The listing builds one solid part. Answer for the finished solid, in the listing's coordinates (mm). A direction names the side the tool comes from. Round coordinates to 2 decimals unless told otherwise and drop trailing zeros. Loops run counter-clockwise (first coordinate to the right, second up) from the corner with the lowest first, then second, coordinate; pieces in that order, holes last. Notation, with made-up numbers: (74.5, 1) - (125.5, 1) arc R16 cw to (125.5, 28) - close; hole circle Ø2 at (-7, 19.25). An arc over 180 degrees is marked (long way). One line per item, written item: value.
```python
from build123d import *

# Parameters (mm, degrees)
SKETCH1_R         = 50.8
EXTRUDE1_DEPTH    = 7.62
SKETCH2_R         = 21.463
EXTRUDE2_DEPTH    = 24.892
SKETCH3_R         = 3.175
EXTRUDE3_DEPTH    = 8.62
CIRPATTERN1_COUNT = 4
FILLET1_R         = 1.154545455
SKETCH4_W         = 79.017488084
SKETCH4_H         = 12.7


with BuildPart() as part:
    # Sketch1 → Extrude1 (new body)
    with BuildSketch(Plane.XY):
        Circle(SKETCH1_R)
    extrude(amount=EXTRUDE1_DEPTH)

    # Sketch2 → Extrude2 (add)
    with BuildSketch(Plane.XY.offset(7.62)):
        Circle(SKETCH2_R)
    extrude(amount=EXTRUDE2_DEPTH)

    # Sketch3 → Extrude3 (cut, through all)
    with BuildSketch(Plane.XY.offset(7.62)):
        with Locations((0, 36.1315)):
            Circle(SKETCH3_R)
    extrude3 = extrude(amount=-EXTRUDE3_DEPTH, mode=Mode.SUBTRACT)

    # CirPattern1: Extrude3 ×4 about axis
    cirpattern1_axis = Axis((0, 0, 0), (0, 0, 1))
    for i in range(1, CIRPATTERN1_COUNT):
        add(extrude3.rotate(cirpattern1_axis, i * 360 / CIRPATTERN1_COUNT), mode=Mode.SUBTRACT)

    # Fillet1
    fillet1_edges = [part.edges().sort_by_distance(p)[0] for p in [
        (-50.8, 0, 7.62),
        (-21.463, 0, 7.62),
        (-21.463, 0, 32.512),
    ]]
    fillet(fillet1_edges, radius=FILLET1_R)

    # Sketch4 → Cut-Revolve1 (revolve, cut)
    with BuildSketch(Plane(origin=(0, 0, 63.5), x_dir=(0, 0, -1), z_dir=(1, 0, 0))):
        with Locations((39.507700489, 6.35)):
            Rectangle(SKETCH4_W, SKETCH4_H)
    revolve(axis=Axis((0, 0, -15.516444531), (0, 0, 1)), mode=Mode.SUBTRACT)


solid = part.part
```
1) For faces 1 (the flat face through (10, -21, 7.62)), 2 (the cylindrical face through (0.688, -33.032, 3.863)), determine the directions among +Z, -Z, +X, -X, +Y, -Y from which every point of the face is accessible in a straight line to the end or side of a thin tool.
Final values:
face 1: +Z
face 2: +Z, -Z
2) A cutting plane is placed at A-A on y = 0. Give the vertices of the cut face in (x, z).
Final values:
outline: (-50.8, 0) - (-39.31, 0) - (-39.31, 7.62) - (-49.65, 7.62) arc R1.15 ccw to (-50.8, 6.47) - close; (-32.96, 0) - (-12.7, 0) - (-12.7, 32.51) - (-20.31, 32.51) arc R1.15 ccw to (-21.46, 31.36) - (-21.46, 8.77) arc R1.15 cw to (-22.62, 7.62) - (-32.96, 7.62) - close; (12.7, 0) - (32.96, 0) - (32.96, 7.62) - (22.62, 7.62) arc R1.15 cw to (21.46, 8.77) - (21.46, 31.36) arc R1.15 ccw to (20.31, 32.51) - (12.7, 32.51) - close; (39.31, 0) - (50.8, 0) - (50.8, 6.47) arc R1.15 ccw to (49.65, 7.62) - (39.31, 7.62) - close
3) A cutting plane is placed at D-D on z = 3. Give the number of separate pieces and of enclosed holes in the cut face, and give its area (3 significant figures).
Final values:
separate pieces: 1
enclosed holes: 5
area: 7,470 mm2
4) For a pull along Y with two mould halves and no side action, classify faces 3 (the flat face through (0, -13, 32.512)), 4 (the cylindrical face through (20.47, 6.45, 19.91)), 5 (the cylindrical face through (-33.032, -0.688, 3.863)) as released by +Y, released by -Y, zero draft, split by the parting line, or undercut.
Final values:
face 3: zero draft
face 4: split by the parting line
face 5: undercut
5) Each of these flat-tipped pins is pushed along its axis until it touches: pin 1 Ø1.5 at (x, y) = (32, 11) entering from +Z; pin 2 Ø12 at (x, z) = (-22.5, 24) entering from +Y; pin 3 Ø5 at (y, z) = (18.5, 11.5) entering from +X. Where does it stop, or does it pass through?
Final values:
pin 1: z = 7.62
pin 2: y = 13.73
pin 3: x = 14.31
6) Consider L1, parallel to Y at x = -0.5, z = 11.5; L2, parallel to X at y = 3, z = 19; L3, parallel to Y at x = 7, z = 2. Determine where each line is inside the solid, lowest interval first.
Final values:
L1: -21.46 to -12.69, 12.69 to 21.46
L2: -21.25 to -12.34, 12.34 to 21.25
L3: -50.32 to -10.6, 10.6 to 50.32
7) A cutting plane is placed at C-C on z = 24. Give the vertices of the cut face in (x, y), and give its area (4 significant figures).
Final values:
outline: circle Ø42.93 at (0, 0); hole circle Ø25.4 at (0, 0)
area: 940.5 mm2
